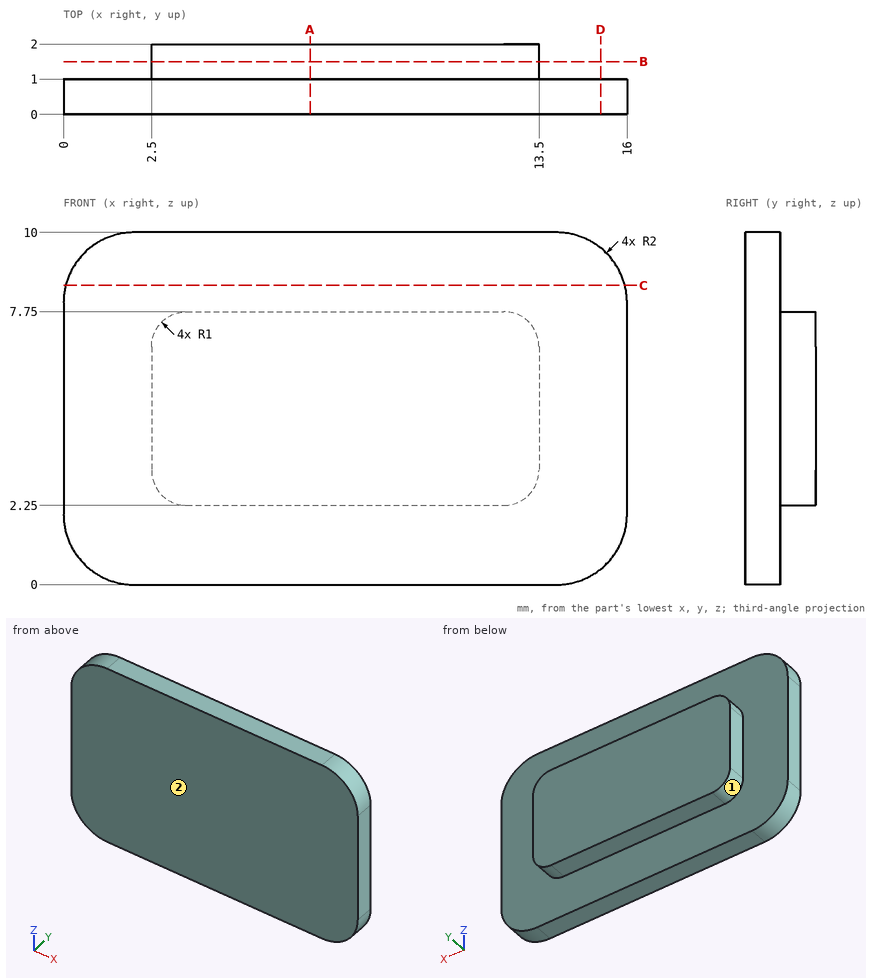
Could you check a few things on this drawing? It's one solid part, dimensions in mm from its lowest x, y, z. A direction names the side the tool comes from. Round coordinates to 2 decimals unless told otherwise and drop trailing zeros. Write each loop counter-clockwise with the first axis right and the second up, starting at its lowest first coordinate (ties: lowest second). Pieces come first, ordered by that corner, then holes.
Q1. If we section it at C-C on z = 8.5: Write out the boundary of the cut face in (x, y), plus the area to 3 significant figures.
Q2. If we section it at A-A on x = 7: Write out the boundary of the cut face in (y, z).
Q3. If we section it at D-D on x = 15.25: Write out the boundary of the cut face in (y, z).
Q4. If we section it at B-B on y = 1.5: Write out the boundary of the cut face in (x, z), plus the area to 3 significant figures.
Q5. Please list where these lines run through material, in increasing order: probe 1 along X at (y, z) = (1.8, 6); probe 2 along Y at (x, z) = (6.5, 2); probe 3 along Z at (x, y) = (9.5, 1.15).
Q6. Which directions (+Z, -Z, +X, -X, +Y, -Y) give clear straight access to the entire face, cutting with the end or side of a thin tool? Please do the marked faces 1 and 2.
Q7. Will these pins go through, and if not, where does the flat tip stop? P1, Ø0.5, axis at x = 10, y = 1.5, coming from the +Z side; P2, Ø0.5, axis at y = 1.5, z = 4, coming from the -X side.
Answer below:
1. outline: (0.06, 0) - (15.94, 0) - (15.94, 1) - (0.06, 1) - close
1. area: 15.9 mm2
2. outline: (0, 0) - (1, 0) - (1, 2.25) - (2, 2.25) - (2, 7.75) - (1, 7.75) - (1, 10) - (0, 10) - close
3. outline: (0, 0.44) - (1, 0.44) - (1, 9.56) - (0, 9.56) - close
4. outline: (2.5, 3.25) arc R1 ccw to (3.5, 2.25) - (12.5, 2.25) arc R1 ccw to (13.5, 3.25) - (13.5, 6.75) arc R1 ccw to (12.5, 7.75) - (3.5, 7.75) arc R1 ccw to (2.5, 6.75) - close
4. area: 59.6 mm2
5. probe 1: x = 2.5 to 13.5
5. probe 2: y = 0 to 1
5. probe 3: z = 2.25 to 7.75
6. face 1: -Z, -X, +Y
6. face 2: +Z, -Z, +X, -X, -Y
7. P1: stops at z = 7.75
7. P2: stops at x = 2.5
